For this review, take the finished solid that the model builds, in its own axes (mm). A direction names the side the tool comes from. Give positions to 0.01 mm unless a question says otherwise; leave off trailing zeros. Loops run counter-clockwise (first coordinate to the right, second up) from the corner with the lowest first, then second, coordinate; pieces in that order, holes last.
```python
from build123d import *

# Parameters (mm, degrees)
EXTRUDE_1_DEPTH = 16
SKETCH_2_W      = 69
SKETCH_2_H      = 5.674471655
EXTRUDE_2_DEPTH = 10


with BuildPart() as part:
    # Sketch 1 → Extrude 1 (new body)
    with BuildSketch(Plane(origin=(0, 0, 0), x_dir=(0, 0, -1), z_dir=(1, 0, 0))):
        with BuildLine():
            Line((-90.049538089, 42.104167983), (-91.224009744, 42.104167983))
            ThreePointArc((-91.224009744, 42.104167983), (-93.345330087, 41.225488326), (-94.224009744, 39.104167983))
            Line((-94.224009744, 39.104167983), (-94.224009744, -20.716289887))
            ThreePointArc((-94.224009744, -20.716289887), (-95.749462998, -25.415251948), (-99.744070854, -28.322202266))
            add(Edge.make_bspline(
                [(-99.744070854, -28.322202266), (-104.134038199, -29.753569103), (-111.139855432, -31.558791211), (-123.096893998, -39.107622001), (-126.096856362, -49.163607245), (-134.645731206, -49.507715511)],
                knots=[0.130050002, 0.130050002, 0.130050002, 0.130050002, 0.418291245, 0.563236081, 0.980272749, 0.980272749, 0.980272749, 0.980272749], degree=3))
            Line((-134.645731206, -49.507715511), (-83.597035684, -49.507715511))
            add(Edge.make_bspline(
                [(-54.064775511, -33.059564163), (-55.113380914, -31.957231859), (-111.694163527, -33.841083074), (-83.597035684, -49.507715511)],
                knots=[0, 0, 0, 0, 1, 1, 1, 1], degree=3))
            add(Edge.make_bspline(
                [(-54.064775511, -33.059564163), (-53.016170109, -31.957231859), (3.564612504, -33.841083074), (-24.532515339, -49.507715511)],
                knots=[0, 0, 0, 0, 1, 1, 1, 1], degree=3))
            Line((-24.532515339, -49.507715511), (26.516180183, -49.507715511))
            add(Edge.make_bspline(
                [(-8.385480169, -28.322202266), (-3.995512823, -29.753569103), (3.010304409, -31.558791211), (14.967342975, -39.107622001), (17.967305339, -49.163607245), (26.516180183, -49.507715511)],
                knots=[0.130050002, 0.130050002, 0.130050002, 0.130050002, 0.418291245, 0.563236081, 0.980272749, 0.980272749, 0.980272749, 0.980272749], degree=3))
            ThreePointArc((-8.385480169, -28.322202266), (-12.380088025, -25.415251948), (-13.905541279, -20.716289887))
            Line((-13.905541279, -20.716289887), (-13.905541279, 39.104167983))
            ThreePointArc((-13.905541279, 39.104167983), (-14.784220936, 41.225488326), (-16.905541279, 42.104167983))
            Line((-16.905541279, 42.104167983), (-18.080012934, 42.104167983))
            ThreePointArc((-18.080012934, 42.104167983), (-20.201333278, 41.225488326), (-21.080012934, 39.104167983))
            Line((-21.080012934, 39.104167983), (-21.080012934, -12.479355565))
            ThreePointArc((-21.080012934, -12.479355565), (-24.008945122, -19.550423377), (-31.080012934, -22.479355565))
            Line((-31.080012934, -22.479355565), (-44.127966284, -22.479355565))
            Line((-44.127966284, -22.479355565), (-54.064775511, -22.479355565))
            Line((-54.064775511, -22.479355565), (-64.001584739, -22.479355565))
            Line((-64.001584739, -22.479355565), (-77.049538089, -22.479355565))
            ThreePointArc((-77.049538089, -22.479355565), (-84.120605901, -19.550423377), (-87.049538089, -12.479355565))
            Line((-87.049538089, -12.479355565), (-87.049538089, 39.104167983))
            ThreePointArc((-87.049538089, 39.104167983), (-87.928217745, 41.225488326), (-90.049538089, 42.104167983))
        make_face()
    extrude(amount=EXTRUDE_1_DEPTH)


with BuildPart() as body_2:
    # Move Body 1: copy of part
    add(part.part.moved(Location((85, 0, 0))))


with BuildPart() as part_1:
    add(part.part)

    add(body_2.part)  # Extrude 2 merges body 2
    # Sketch 2 → Extrude 2 (add)
    with BuildSketch(Plane(origin=(0, 0, 0), x_dir=(1, 0, 0), z_dir=(0, 1, 0))):
        with Locations((50.5, -91.386773917)):
            Rectangle(SKETCH_2_W, SKETCH_2_H)
        with Locations((50.5, -16.742777107)):
            Rectangle(SKETCH_2_W, SKETCH_2_H)
    extrude(amount=EXTRUDE_2_DEPTH)


solid = part_1.part
```
Q1. Consider section C-C on y = 24. Give the boundary of the cut face in (x, z), plus the area to 3 significant figures.
Answers:
outline: (0, 13.91) - (16, 13.91) - (16, 21.08) - (0, 21.08) - close; (0, 87.05) - (16, 87.05) - (16, 94.22) - (0, 94.22) - close; (85, 13.91) - (101, 13.91) - (101, 21.08) - (85, 21.08) - close; (85, 87.05) - (101, 87.05) - (101, 94.22) - (85, 94.22) - close
area: 459 mm2
Q2. For pin 1 Ø4 at (x, z) = (86, 53) entering from -Y; pin 2 Ø8 at (x, y) = (89.5, 22) entering from +Z; pin 3 Ø4.5 at (x, z) = (45.5, 92.5) entering from -Y, all flat-tipped, find the tip position at first contact; note any pin that passes through.
Answers:
pin 1: stops at y = -33.06
pin 2: stops at z = 94.22
pin 3: stops at y = 0
Q3. For probe 1 along Z at (x, y) = (88.5, -8); probe 2 along X at (y, z) = (-42, 117); probe 3 along Z at (x, y) = (38.5, 7.5), list the stretches that pass through material, from the lowest coordinate up.
Answers:
probe 1: z = 13.91 to 21.08, 87.05 to 94.22
probe 2: x = 0 to 16, 85 to 101
probe 3: z = 13.91 to 19.58, 88.55 to 94.22
Q4. Machinability: for faces 1 (the flat face through (50, 5, 19.58)), 2 (the flat face through (50, 9, 13.906)), 3 (the flat face through (50, 10, 91)), 4 (the flat face through (49.8, 9.6, 94.224)), which of the approach directions +Z, -Z, +X, -X, +Y, -Y give a long, thin tool a straight path to every point of the face, cutting with its end or side? Answer none if there is none.
Answers:
face 1: +Y, -Y
face 2: -Z, +X, -X, +Y
face 3: +Z, -Z, +Y
face 4: +Z, +X, -X, +Y
Q5. Consider section B-B on y = 3. Give the boundary of the cut face in (x, z), plus the area to 3 significant figures.
Answers:
outline: (0, 13.91) - (101, 13.91) - (101, 21.08) - (85, 21.08) - (85, 19.58) - (16, 19.58) - (16, 21.08) - (0, 21.08) - close; (0, 87.05) - (16, 87.05) - (16, 88.55) - (85, 88.55) - (85, 87.05) - (101, 87.05) - (101, 94.22) - (0, 94.22) - close
area: 1,240 mm2
Q6. Mouldability with a two-part tool opening along Z and no side actions: class faces 5 (the cylindrical face through (92.89, -25.47, 12.34)), 6 (the flat face through (8, -49.508, -1)), 7 (the cylindrical face through (92.89, -19.47, 23.93)), 8 (the cylindrical face through (92.89, -19.63, 84.04)) as +Z half, -Z half, draft (parallel to the pull), parting line (faces both ways), or undercut.
Answers:
face 5: -Z half
face 6: draft
face 7: undercut
face 8: undercut
Q7. Consider section A-A on x = 69.5. Give the boundary of the cut face in (y, z), plus the area to 3 significant figures.
Answers:
outline: (0, 13.91) - (10, 13.91) - (10, 19.58) - (0, 19.58) - close; (0, 88.55) - (10, 88.55) - (10, 94.22) - (0, 94.22) - close
area: 113 mm2
